from build123d import *

# Parameters (mm, degrees)
SKETCH1_W               = 112
SKETCH1_H               = 58
BOSS_EXTRUDE1_DEPTH     = 0.8
SKETCH2_W               = 112
SKETCH2_H               = 58
SKETCH2_W_2             = 110
SKETCH2_H_2             = 56
BOSS_EXTRUDE2_DEPTH     = 28
SKETCH3_R               = 1.75
CUT_EXTRUDE1_DEPTH      = 28
BOSS_EXTRUDE3_START     = 2
SKETCH4_R               = 3.25
SKETCH4_R_2             = 1.75
BOSS_EXTRUDE3_DEPTH     = 2
CUT_EXTRUDE2_DEPTH      = 2
CUT_EXTRUDE3_DEPTH      = 72
BOSS_EXTRUDE4_DEPTH     = 28.8
SKETCH8_W               = 11.5
SKETCH8_H               = 1.5
CUT_EXTRUDE4_DEPTH      = 70
CUT_EXTRUDE5_DEPTH      = 70
CUT_EXTRUDE5_DEPTH_BACK = 70
SKETCH9_W               = 112
SKETCH9_H               = 28
SKETCH10_W              = 8.327989843
SKETCH10_H              = 7.445097605
SKETCH10_W_2            = 5.355096577
SKETCH10_H_2            = 5.953712533
SKETCH10_W_3            = 11.410895322
SKETCH10_H_3            = 5.715079946
SKETCH10_W_4            = 8.730278995
SKETCH10_H_4            = 7.857983818
BOSS_EXTRUDE5_DEPTH     = 0.8
SKETCH11_W              = 106.4
SKETCH11_H              = 52.4
BOSS_EXTRUDE6_DEPTH     = 3
SKETCH12_W              = 10.5
SKETCH12_H              = 1
BOSS_EXTRUDE7_DEPTH     = 1
SKETCH13_W              = 10.5
SKETCH13_H              = 1
BOSS_EXTRUDE8_DEPTH     = 1
SKETCH14_W              = 1.3
SKETCH14_H              = 4
BOSS_EXTRUDE9_DEPTH     = 15
SKETCH15_W              = 3
SKETCH15_H              = 1.5
CUT_EXTRUDE6_DEPTH      = 70
FILLET1_R               = 1


with BuildPart() as part:
    # Sketch1 → Boss-Extrude1 (new body)
    with BuildSketch(Plane(origin=(0, 0, 0), x_dir=(1, 0, 0), z_dir=(0, 1, 0))):
        Rectangle(SKETCH1_W, SKETCH1_H)
    extrude(amount=BOSS_EXTRUDE1_DEPTH)

    # Sketch2 → Boss-Extrude2 (add)
    with BuildSketch(Plane(origin=(0, 0.8, 0), x_dir=(1, 0, 0), z_dir=(0, 1, 0))):
        Rectangle(SKETCH2_W, SKETCH2_H)
        Rectangle(SKETCH2_W_2, SKETCH2_H_2, mode=Mode.SUBTRACT)
    extrude(amount=BOSS_EXTRUDE2_DEPTH)

    # Sketch3 → Cut-Extrude1 (cut)
    with BuildSketch(Plane(origin=(0, 0.8, 0), x_dir=(1, 0, 0), z_dir=(0, 1, 0))):
        with Locations(Location((-36, 25.5, 0), (0, 0, 270))):
            Circle(SKETCH3_R)
        with Locations(Location((-36, -25.5, 0), (0, 0, 270))):
            Circle(SKETCH3_R)
        with Locations(Location((45.5, 25.5, 0), (0, 0, 270))):
            Circle(SKETCH3_R)
        with Locations(Location((45.5, -25.5, 0), (0, 0, 270))):
            Circle(SKETCH3_R)
    extrude(amount=-CUT_EXTRUDE1_DEPTH, mode=Mode.SUBTRACT)

    # Sketch4 → Boss-Extrude3 (add)
    # profile 1 of 4: a face of its own
    with BuildSketch(Plane(origin=(0, 0.8, 0), x_dir=(1, 0, 0), z_dir=(0, 1, 0)).offset(BOSS_EXTRUDE3_START)):
        with Locations((-36, 25.5)):
            Circle(SKETCH4_R)
        with Locations(Location((-36, 25.5, 0), (0, 0, 270))):
            Circle(SKETCH4_R_2, mode=Mode.SUBTRACT)
    # profile 2 of 4: a face of its own
    with BuildSketch(Plane(origin=(0, 0.8, 0), x_dir=(1, 0, 0), z_dir=(0, 1, 0)).offset(BOSS_EXTRUDE3_START)):
        with Locations((45.5, 25.5)):
            Circle(SKETCH4_R)
        with Locations(Location((45.5, 25.5, 0), (0, 0, 270))):
            Circle(SKETCH4_R_2, mode=Mode.SUBTRACT)
    # profile 3 of 4: a face of its own
    with BuildSketch(Plane(origin=(0, 0.8, 0), x_dir=(1, 0, 0), z_dir=(0, 1, 0)).offset(BOSS_EXTRUDE3_START)):
        with Locations((-36, -25.5)):
            Circle(SKETCH4_R)
        with Locations(Location((-36, -25.5, 0), (0, 0, 270))):
            Circle(SKETCH4_R_2, mode=Mode.SUBTRACT)
    # profile 4 of 4: a face of its own
    with BuildSketch(Plane(origin=(0, 0.8, 0), x_dir=(1, 0, 0), z_dir=(0, 1, 0)).offset(BOSS_EXTRUDE3_START)):
        with Locations((45.5, -25.5)):
            Circle(SKETCH4_R)
        with Locations(Location((45.5, -25.5, 0), (0, 0, 270))):
            Circle(SKETCH4_R_2, mode=Mode.SUBTRACT)
    extrude(amount=-BOSS_EXTRUDE3_DEPTH)

    # Sketch5 → Cut-Extrude2 (cut)
    with BuildSketch(Plane(origin=(-55, 0, 0), x_dir=(0, 0, -1), z_dir=(1, 0, 0))):
        with BuildLine():
            Line((-10.5, 28.8), (-10.5, 10.8))
            ThreePointArc((-10.5, 10.8), (-8, 8.3), (-5.5, 10.8))
            Line((-5.5, 10.8), (-5.5, 28.8))
            Line((-5.5, 28.8), (-10.5, 28.8))
        make_face()
    extrude(amount=-CUT_EXTRUDE2_DEPTH, mode=Mode.SUBTRACT)

    # Sketch6 → Cut-Extrude3 (cut)
    with BuildSketch(Plane.XY.offset(29)):
        with BuildLine():
            Line((34.5, 25.8), (34.5, 28.8))
            Line((34.5, 28.8), (37.5, 28.8))
            Line((37.5, 28.8), (37.5, 25.8))
            ThreePointArc((37.5, 25.8), (36, 24.3), (34.5, 25.8))
        make_face()
    extrude(amount=-CUT_EXTRUDE3_DEPTH, mode=Mode.SUBTRACT)

    # Sketch7 → Boss-Extrude4 (add)
    with BuildSketch(Plane.XZ):
        Polygon((-41, 29), (-38, 32), (-34, 32), (-31, 29), align=None)
        Polygon((40.5, 29), (43.5, 32), (47.5, 32), (50.5, 29), align=None)
        Polygon((-41, -29), (-38, -32), (-34, -32), (-31, -29), align=None)
        Polygon((40.5, -29), (43.5, -32), (47.5, -32), (50.5, -29), align=None)
    extrude(amount=-BOSS_EXTRUDE4_DEPTH)

    # Sketch8 → Cut-Extrude4 (cut)
    with BuildSketch(Plane.XY.offset(29)):
        with Locations((4.75, 26.55)):
            Rectangle(SKETCH8_W, SKETCH8_H)
    extrude(amount=-CUT_EXTRUDE4_DEPTH, mode=Mode.SUBTRACT)

    # Sketch9 → Cut-Extrude5 (cut, two sides: drawn at the far end of the back side and taken through both)
    with BuildSketch(Plane.XY.offset(29).offset(-CUT_EXTRUDE5_DEPTH_BACK)):
        with Locations((0, 14.8)):
            Rectangle(SKETCH9_W, SKETCH9_H)
    extrude(amount=CUT_EXTRUDE5_DEPTH + CUT_EXTRUDE5_DEPTH_BACK, mode=Mode.SUBTRACT)

    # Sketch10 → Boss-Extrude5 (add)
    with BuildSketch(Plane(origin=(0, 0.8, 0), x_dir=(1, 0, 0), z_dir=(0, 1, 0))):
        with Locations((-35.349106924, 23.952885498)):
            Rectangle(SKETCH10_W, SKETCH10_H)
        with Locations((45.232488371, 24.698578034)):
            Rectangle(SKETCH10_W_2, SKETCH10_H_2)
        with Locations((-36.890559663, -24.651256065)):
            Rectangle(SKETCH10_W_3, SKETCH10_H_3)
        with Locations((45.075573152, -24.28226276)):
            Rectangle(SKETCH10_W_4, SKETCH10_H_4)
    extrude(amount=-BOSS_EXTRUDE5_DEPTH)

    # Sketch11 → Boss-Extrude6 (add)
    with BuildSketch(Plane(origin=(0, 0.8, 0), x_dir=(1, 0, 0), z_dir=(0, 1, 0))):
        Polygon((-51.704605873, 27.7), (-54.7, 27.7), (-54.7, 25.360609515), (-54.7, -24.546387496), (-54.7, -27.7), (-52.806207703, -27.7), (50.795370915, -27.7), (54.7, -27.7), (54.7, -25.222572544), (54.7, 24.684424467), (54.7, 27.7), (51.896972744, 27.7), align=None)
        Rectangle(SKETCH11_W, SKETCH11_H, mode=Mode.SUBTRACT)
    extrude(amount=BOSS_EXTRUDE6_DEPTH)

    # Sketch12 → Boss-Extrude7 (add)
    with BuildSketch(Plane.XY.offset(27.7)):
        with Locations((4.75, 3.3)):
            Rectangle(SKETCH12_W, SKETCH12_H)
    extrude(amount=BOSS_EXTRUDE7_DEPTH)

    # Sketch13 → Boss-Extrude8 (add)
    with BuildSketch(Plane(origin=(0, 0, -27.7), x_dir=(-1, 0, 0), z_dir=(0, 0, -1))):
        with Locations((-4.75, 3.3)):
            Rectangle(SKETCH13_W, SKETCH13_H)
    extrude(amount=BOSS_EXTRUDE8_DEPTH)

    # Sketch14 → Boss-Extrude9 (add)
    with BuildSketch(Plane(origin=(0, 0.8, 0), x_dir=(1, 0, 0), z_dir=(0, 1, 0))):
        with Locations((-55.35, 8)):
            Rectangle(SKETCH14_W, SKETCH14_H)
    extrude(amount=BOSS_EXTRUDE9_DEPTH)

    # Sketch15 → Cut-Extrude6 (cut)
    with BuildSketch(Plane.XY.offset(27.7)):
        with Locations((36, 3.05)):
            Rectangle(SKETCH15_W, SKETCH15_H)
    extrude(amount=-CUT_EXTRUDE6_DEPTH, mode=Mode.SUBTRACT)

    # Fillet1
    fillet1_edges = [part.edges().sort_by_distance(p)[0] for p in [
        (37.5, 2.3, 26.95),
        (37.5, 2.3, -26.95),
        (34.5, 2.3, 26.95),
        (34.5, 2.3, -26.95),
    ]]
    fillet(fillet1_edges, radius=FILLET1_R)


solid = part.part
Check sheet for the modelled part. Datum: model origin and axes. Units: mm. A direction names the side the tool comes from. Round coordinates to 2 decimals unless told otherwise and drop trailing zeros. Write each loop counter-clockwise with the first axis right and the second up, starting at its lowest first coordinate (ties: lowest second). Pieces come first, ordered by that corner, then holes. Notation, with made-up numbers: (59.25, 52.25) - (70.25, 52.25) arc R31 ccw to (70.25, 87.25) - close; hole circle Ø9 at (54, -40). An arc over 180 degrees is marked (long way). Return JSON: item names as keys, results as strings.
Q1. Cross-section at A-A (x = -12). Record the boundary of the cut face in (y, z), then the cut area to 3 significant figures.
Returned:
{"outline": "(0, -29) - (0.8, -29) - (0.8, -27.7) - (3.8, -27.7) - (3.8, -26.2) - (0.8, -26.2) - (0.8, 26.2) - (3.8, 26.2) - (3.8, 27.7) - (0.8, 27.7) - (0.8, 29) - (0, 29) - close", "area": "55.4 mm²"}
Q2. Depth check by flat-ended pin: P1, Ø3.5, axis at y = 2, z = -21.5, coming from the -X side; P2, Ø5, axis at x = -31.5, z = -11, coming from the +Y side; P3, Ø0.9, axis at x = 5.5, y = 2, coming from the +Z side; P4, Ø2.5, axis at x = -3, y = 2, coming from the -Z side. Enter the tip coordinate at first touch or a pass-through.
Returned:
{"P1": "stops at x = -56", "P2": "stops at y = 0.8", "P3": "stops at z = 27.7", "P4": "stops at z = -29"}
Q3. Cross-section at C-C (y = 7). Record the boundary of the cut face in (x, z).
Returned:
{"outline": "(-56, -10) - (-54.7, -10) - (-54.7, -6) - (-56, -6) - close"}
Q4. Draft check along X on faces 4 (the flat face through (-32.5, 0.4, 30.5)), 5 (the flat face through (0, 0.8, 28)), 6 (the flat face through (-56, 5.5, -6.3)). Enter one of: released by +X, released by -X, zero draft, split by the parting line, or undercut.
Returned:
{"face 4": "undercut", "face 5": "zero draft", "face 6": "released by -X"}
Q5. Cross-section at B-B (z = 1.5). Record the boundary of the cut face in (x, y), then the cut area to 3 significant figures.
Returned:
{"outline": "(-56, 0) - (56, 0) - (56, 0.8) - (54.7, 0.8) - (54.7, 3.8) - (53.2, 3.8) - (53.2, 0.8) - (-53.2, 0.8) - (-53.2, 3.8) - (-54.7, 3.8) - (-54.7, 0.8) - (-56, 0.8) - close", "area": "98.6 mm²"}
Q6. Access from +Z, -Z, +X, -X, +Y, -Y to the whole of each face (thin tool, end or side, straight path). Record for faces 1 (the flat face through (53.2, 2, 0)), 2 (the flat face through (-54.7, 10, -8)), 3 (the flat face through (-54.7, 2, 11)).
Returned:
{"face 1": "+Y", "face 2": "+Z, -Z, +X, +Y", "face 3": "+Z, -X, +Y"}
Q7. Scan lines: L1, parallel to X at y = 2.5, z = 10.5; L2, parallel to Z at x = 27, y = 1.5; L3, parallel to Y at x = 17, z = -14. Record each from-to range of solid material in increasing order. Write a range as from..to.
Returned:
{"L1": "x = -54.7..-53.2, 53.2..54.7", "L2": "z = -27.7..-26.2, 26.2..27.7", "L3": "y = 0..0.8"}
